Part model, mm, in its own coordinate system. Face numbers are marked on the shaded views. Round coordinates to 2 decimals unless told otherwise and drop trailing zeros. Loops run counter-clockwise (first coordinate to the right, second up) from the corner with the lowest first, then second, coordinate; pieces in that order, holes last.
1) Band-saw the part on B-B, the plane x = 14.5. Write the cut outline in (y, z) (3 decimals), then the cut area to 3 significant figures.
2) Mould opens along Z. For the marked faces 1, 2, 3 and 4 say: +Z half, -Z half, draft (parallel to the pull), parting line (faces both ways), or undercut.
3) Band-saw the part on A-A, the plane x = 23. Write the cut outline in (y, z), then the cut area to 3 significant figures.
4) Drop flat-ended pins along their axis: P1, Ø2, axis at y = 75.5, z = 271.5, coming from the -X side; P2, Ø8, axis at x = 23.5, y = 61, coming from the -Z side; P3, Ø12, axis at x = -11.5, z = 297.5, coming from the -Y side. Give the stop position or say it passes through.
5) Probe line 1 (Z direction, x = -2, y = 76); line 2 (Z direction, x = 20, y = 50); line 3 (X direction, y = 68.5, z = 283). List the from-to ranges inside material, lowest first.
from build123d import *

# Parameters (mm, degrees)
SKETCH11_R               = 17.249999999999545
BOSS_EXTRUDE2_DEPTH      = 1
BOSS_EXTRUDE1_DEPTH      = 17.25
BOSS_EXTRUDE1_DEPTH_BACK = 17.25
CUT_EXTRUDE1_START       = -14.25
SKETCH8_W                = 52.49999999999948
SKETCH8_H                = 37.00000000000014
CUT_EXTRUDE1_DEPTH       = 28.5
M2_5_CLEARANCE_HOLE1_D   = 2.7
CUT_EXTRUDE2_DEPTH       = 287.9075330139404
MOVE_FACE1_BY            = 0.05
MOVE_FACE1_2_BY          = 0.05
FILLET3_R                = 1
SKETCH13_R               = 10.949999999999743
CUT_EXTRUDE3_DEPTH       = 287.92025460072404
CHAMFER1_SIZE            = 0.5
CHAMFER2_SIZE            = 1.5


# Read off the part's stored shape, not the designer's step: Glue_In_Plug
with BuildPart() as part:
    # Glue_In_Plug outline → Glue_In_Plug (revolve)
    with BuildSketch(Plane(origin=(0, 176.776695297, 176.776695297), x_dir=(1, 0, 0), z_dir=(0, 0.707106781186551, 0.707106781186544))):
        with BuildLine():
            Line((12.95, -137.75), (10.95, -137.75))
            Line((10.95, -137.75), (10.95, -156.75))
            Line((10.95, -156.75), (15, -156.75))
            Line((15, -156.75), (15, -155.75))
            Line((15, -155.75), (12.95, -155.75))
            Line((12.95, -155.75), (12.95, -151.482050808))
            ThreePointArc((12.95, -151.482050808), (12.2, -150.183012702), (12.95, -148.883974596))
            Line((12.95, -148.883974596), (12.95, -144.616025404))
            ThreePointArc((12.95, -144.616025404), (12.2, -143.316987298), (12.95, -142.017949192))
            Line((12.95, -142.017949192), (12.95, -137.75))
        make_face()
    revolve(axis=Axis((0, 176.776695297, 176.776695297), (0, 0.707106781186544, -0.707106781186551)))

    # Sketch11 → Boss-Extrude2 (add)
    with BuildSketch(Plane(origin=(0, -110.13188116980581, 110.13188116980702), x_dir=(1, 0, 0), z_dir=(0, 0.7071067811865438, -0.7071067811865513))):
        with Locations(Location((0, -250, 0), (0, 0, 270))):
            Circle(SKETCH11_R)
    extrude(amount=-BOSS_EXTRUDE2_DEPTH)

    # Sketch6 → Boss-Extrude1 (add, two sides: drawn at the far end of the back side and taken through both)
    with BuildSketch(Plane(origin=(0, 176.7766952966368, 176.77669529663697), x_dir=(-1, 0, 0), z_dir=(0, -0.7071067811865477, -0.7071067811865475)).offset(-BOSS_EXTRUDE1_DEPTH_BACK)):
        with BuildLine():
            Line((-32, -156.75000000000077), (-32.00000000000001, -173.7500000000009))
            ThreePointArc((-32.00000000000001, -173.7500000000009), (-30.828427124746195, -176.5784271247471), (-27.999999999999996, -177.75000000000088))
            Line((-27.999999999999996, -177.75000000000088), (-4.0000000000000036, -177.75000000000088))
            ThreePointArc((-4.0000000000000036, -177.75000000000088), (-2.5528006726860175, -177.47902321084604), (-1.3016800588632904, -176.7028070535119))
            Line((-1.3016800588632904, -176.7028070535119), (17.249999999999545, -159.75000000000082))
            Line((17.249999999999545, -159.75000000000082), (17.249999999999545, -156.75000000000077))
            Line((17.249999999999545, -156.75000000000077), (-32, -156.75000000000077))
        make_face()
    extrude(amount=BOSS_EXTRUDE1_DEPTH + BOSS_EXTRUDE1_DEPTH_BACK)

    # Sketch8 → Cut-Extrude1 (cut)
    with BuildSketch(Plane(origin=(0, 176.7766952966368, 176.77669529663697), x_dir=(-1, 0, 0), z_dir=(0, -0.7071067811865477, -0.7071067811865475)).offset(CUT_EXTRUDE1_START)):
        with Locations((-9.000000000000195, -178.2500000000009)):
            Rectangle(SKETCH8_W, SKETCH8_H)
    extrude(amount=CUT_EXTRUDE1_DEPTH, mode=Mode.SUBTRACT)

    # M2.5 Clearance Hole1 (through all)
    with Locations(Plane(origin=(0, 188.97428727210456, 188.9742872721045), x_dir=(1, 0, 0), z_dir=(0, 0.7071067811865476, 0.7071067811865476))):
        with Locations((4, -173.75), (28, -173.75)):
            Hole(M2_5_CLEARANCE_HOLE1_D / 2)

    # Sketch12 → Cut-Extrude2 (cut, through all)
    with BuildSketch(Plane(origin=(0, -110.838987950992, 110.83898795099203), x_dir=(1, 7e-16, -7e-16), z_dir=(0, 0.7071067811865476, -0.7071067811865476))):
        with BuildLine():
            Line((-17.249999999999545, -250.00000000000088), (-17.249999999999545, -267.24999999999955))
            Line((-17.249999999999545, -267.24999999999955), (0, -267.24999999999955))
            ThreePointArc((-6.1e-16, -267.24999999999955), (-12.197591975467768, -262.1975919754684), (-17.249999999999538, -250.00000000000088))
        make_face()
        with BuildLine():
            Line((-17.249999999999545, -232.7499999999995), (-17.249999999999545, -250.00000000000088))
            ThreePointArc((-17.24999999999954, -250.00000000000088), (-12.197591975468656, -237.80240802453167), (0, -232.7499999999995))
            Line((0, -232.7499999999995), (-17.249999999999545, -232.7499999999995))
        make_face()
    extrude(amount=-CUT_EXTRUDE2_DEPTH, mode=Mode.SUBTRACT)

    # Move Face1: a face moved inward by 0.05
    extrude(part.faces().sort_by_distance((12.658853914, 47.847886018, 285.552961311))[0], amount=MOVE_FACE1_BY, dir=(0, -0.707106781, -0.707106781), mode=Mode.SUBTRACT)

    # Move Face1 2: a face moved inward by 0.05
    extrude(part.faces().sort_by_distance((12.658853914, 68.000429282, 305.705504575))[0], amount=MOVE_FACE1_2_BY, dir=(0, 0.707106781, 0.707106781), mode=Mode.SUBTRACT)

    # Fillet3
    fillet3_edges = [part.edges().sort_by_distance(p)[0] for p in [
        (-9.647408978600675, 71.47175017032276, 302.3048943648676),
        (-9.647408978601732, 51.24849622840657, 282.0816404229506),
    ]]
    fillet(fillet3_edges, radius=FILLET3_R)

    # Sketch13 → Cut-Extrude3 (cut, through all)
    with BuildSketch(Plane(origin=(0, -110.13188116980584, 110.13188116980702), x_dir=(1, 0, 0), z_dir=(0, 0.7071067811865438, -0.7071067811865512))):
        with Locations(Location((0, -250.0000000000001, 0), (0, 0, 90))):
            Circle(SKETCH13_R)
    extrude(amount=-CUT_EXTRUDE3_DEPTH, mode=Mode.SUBTRACT)

    # Chamfer1
    chamfer1_edges = [part.edges().sort_by_distance(p)[0] for p in [
        (-2.01e-15, 71.55920625607847, 297.4798228451817),
    ]]
    chamfer(chamfer1_edges, length=CHAMFER1_SIZE)

    # Chamfer2
    chamfer2_edges = [part.edges().sort_by_distance(p)[0] for p in [
        (32, 65.93770734564494, 287.6156832476289),
    ]]
    chamfer(chamfer2_edges, length=CHAMFER2_SIZE)


solid = part.part
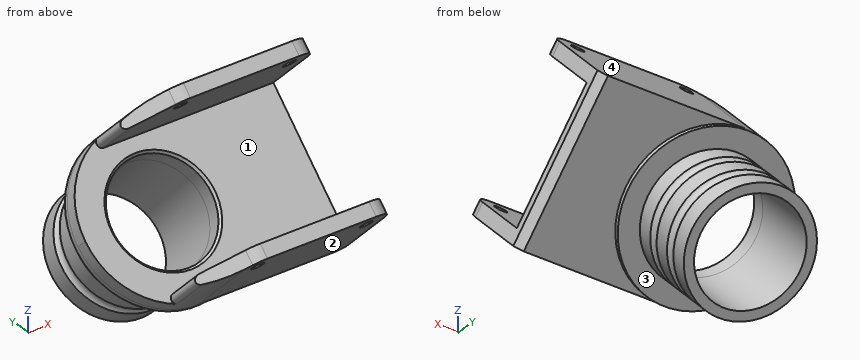
Reported:
1. outline: (38.891, 290.267) - (53.74, 275.418) - (59.33, 281.008) - (60.038, 280.301) - (73.252, 293.516) - (72.545, 294.223) - (78.135, 299.813) - (63.286, 314.663) - (61.2, 312.577) - (73.928, 299.849) - (53.705, 279.625) - (40.977, 292.353) - close
1. area: 228 mm2
2. face 1: undercut
2. face 2: -Z half
2. face 3: undercut
2. face 4: +Z half
3. outline: (38.89, 290.27) - (53.74, 275.42) - (78.14, 299.81) - (63.29, 314.66) - (61.2, 312.58) - (73.93, 299.85) - (53.7, 279.63) - (40.98, 292.35) - close
3. area: 210 mm2
4. P1: stops at x = -12.43
4. P2: stops at z = 278.68
4. P3: stops at y = 65.58
5. line 1: z = 292.78 to 295.65, 296.26 to 301.78
5. line 2: z = 279.16 to 283.33
5. line 3: x = -12.87 to -10.85, 10.85 to 12.87
